Check sheet for the drawn part. Datum: minimum x, y, z corner. Units: mm. A direction names the side the tool comes from. Coordinates: 2 decimals unless noted, no trailing zeros. Write each loop counter-clockwise with the first axis right and the second up, starting at its lowest first coordinate (ties: lowest second). Pieces come first, ordered by that corner, then holes. Notation, with made-up numbers: (36, 87) -> (78, 87) arc R4 ccw to (78, 94) -> close; hole circle Ø11 at (-35.75, -0.75). An arc over 180 degrees is marked (long way). Answer in a Markdown table with one row per item. Add a question column.
Q1. Section check A-A, the plane y = 4.75. Record the boundary of the cut face in (x, z), and give its area (3 significant figures).
Q2. Section check B-B, the plane x = 7.75. Record the boundary of the cut face in (y, z), and give its area (3 significant figures).
Q3. Thickness scan on line 1 (X direction, y = 8.5, z = 3.75); line 2 (Z direction, x = 6.75, y = 6.75); line 3 (X direction, y = 4.5, z = 4.5). Record the ranges inside material, lowest first.
Q4. Tool access check on the marked faces 1, 2 and 3. Record the directions out of +Z, -Z, +X, -X, +Y, -Y that give a thin tool (end or side, any length) a straight path to the whole face; none if there is none.
Q5. Gauge pin test, flat ends, axial feed: P1, Ø4, axis at x = 8.5, z = 3, coming from the +Y side; P2, Ø3, axis at x = 9.5, z = 2.5, coming from the +Y side; P3, Ø3, axis at x = 10, z = 3, coming from the -Y side; P4, Ø4, axis at x = 5.5, y = 4.5, coming from the +Z side. Record the tip position at first contact, or that the pin passes through.
Q6. Release check for a two-part mould opening along Z. For the marked faces 4, 5 and 6 record: pulls with the +Z half, pulls with the -Z half, needs draft (parallel to the pull), parting line crosses it, or undercut.
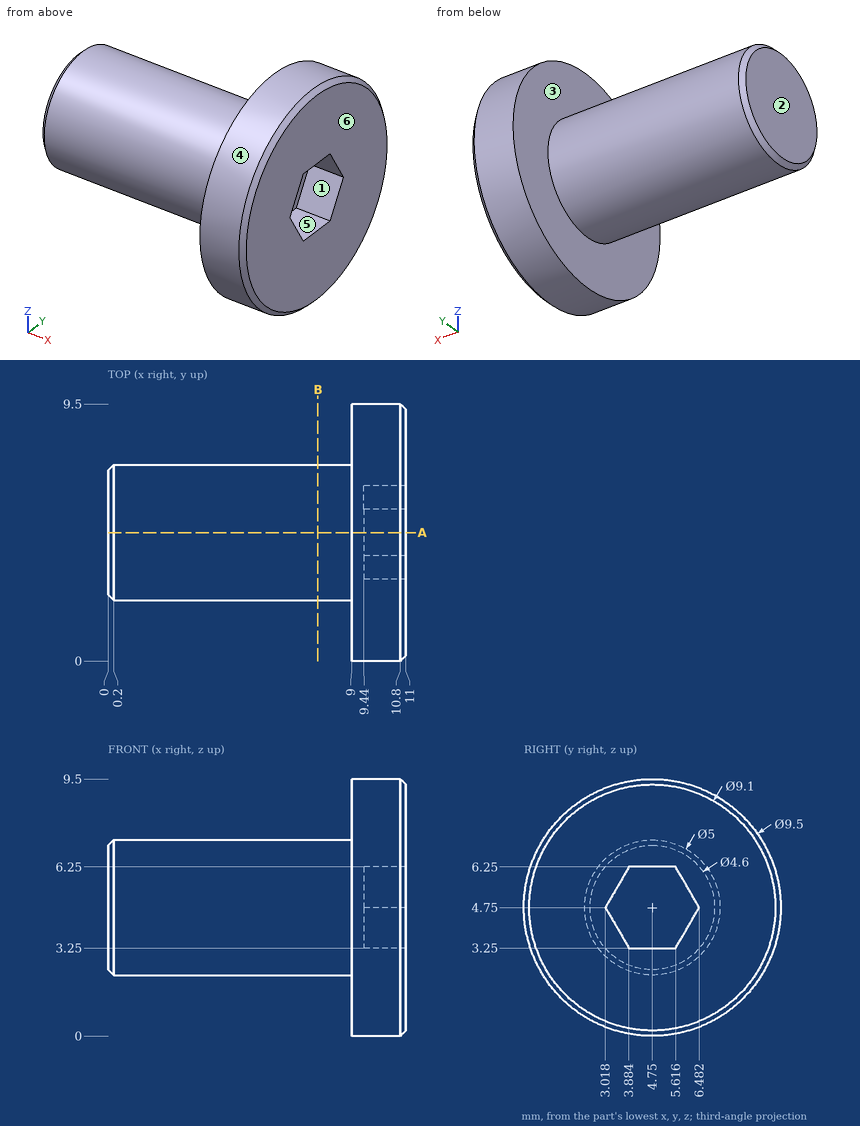
Calculated:
| question | item | result |
|---|---|---|
| 1 | outline | (0, 2.45) -> (0.2, 2.25) -> (9, 2.25) -> (9, 0) -> (10.8, 0) -> (11, 0.2) -> (11, 3.25) -> (9.44, 3.25) -> (9.44, 6.25) -> (11, 6.25) -> (11, 9.3) -> (10.8, 9.5) -> (9, 9.5) -> (9, 7.25) -> (0.2, 7.25) -> (0, 7.05) -> close |
| 1 | area | 59.2 mm² |
| 2 | outline | circle Ø5 at (4.75, 4.75) |
| 2 | area | 19.6 mm² |
| 3 | line 1 | x = 9 to 11 |
| 3 | line 2 | z = 3.25 to 6.25 |
| 3 | line 3 | x = 0 to 9.44 |
| 4 | face 1 | +X |
| 4 | face 2 | +Z, -Z, -X, +Y, -Y |
| 4 | face 3 | -X |
| 5 | P1 | stops at y = 9.5 |
| 5 | P2 | stops at y = 9.44 |
| 5 | P3 | stops at y = 0.01 |
| 5 | P4 | stops at z = 7.25 |
| 6 | face 4 | parting line crosses it |
| 6 | face 5 | undercut |
| 6 | face 6 | needs draft |
